Read the model definition and answer for the solid it produces. Units are mm, in the model's axes. A direction names the side the tool comes from. Coordinates: 2 decimals unless noted, no trailing zeros. Write each loop counter-clockwise with the first axis right and the second up, starting at its lowest first coordinate (ties: lowest second). Pieces come first, ordered by that corner, then holes. Notation, with made-up numbers: (89.25, 4.25) - (133.25, 4.25) arc R27 ccw to (133.25, 29.25) - close; hole circle Ø6 at (-22.75, -10.5). An arc over 180 degrees is marked (long way). Use a Markdown table: item, result.
from build123d import *

# Parameters (mm, degrees)
BOSS_EXTRUDE1_DEPTH = 3.9
SKETCH1_6_R         = 2.1
CUT_EXTRUDE1_DEPTH  = 1.6


with BuildPart() as part:
    # Sketch1 → Boss-Extrude1 (new body)
    with BuildSketch(Plane(origin=(0, 0, 0), x_dir=(1, 0, 0), z_dir=(0, 1, 0))):
        with BuildLine():
            Line((-105.9, 60.929794432), (-105.9, -60.929794385))
            ThreePointArc((-105.9, -60.929794385), (-105.050609665, -62.980404051), (-103, -63.829794385))
            Line((-103, -63.829794385), (2, -63.829794385))
            Line((2, -63.829794385), (2, 63.829794385))
            Line((2, 63.829794385), (-103, 63.829794385))
            ThreePointArc((-103, 63.829794385), (-105.050609649, 62.980404067), (-105.9, 60.929794432))
        make_face()
    extrude(amount=BOSS_EXTRUDE1_DEPTH)

    # Sketch1_6 → Cut-Extrude1 (cut)
    with BuildSketch(Plane(origin=(0, 0, 0), x_dir=(1, 0, 0), z_dir=(0, 1, 0))):
        with Locations(Location((-5, 60.929794385, 0), (0, 0, 270))):
            Circle(SKETCH1_6_R)
        with Locations(Location((-103, -60.929794385, 0), (0, 0, 270))):
            Circle(SKETCH1_6_R)
        with Locations(Location((-5, -60.929794385, 0), (0, 0, 270))):
            Circle(SKETCH1_6_R)
        with Locations(Location((-103, 60.929794385, 0), (0, 0, 270))):
            Circle(SKETCH1_6_R)
    extrude(amount=CUT_EXTRUDE1_DEPTH, mode=Mode.SUBTRACT)


solid = part.part
(1) Each of these flat-tipped pins is pushed along its axis until it touches: P1, Ø3.5, axis at x = -102, z = 61, coming from the -Y side; P2, Ø1.3, axis at x = -103, z = -61.5, coming from the -Y side. Where does it stop, or does it pass through?
Report:
| item | result |
|---|---|
| P1 | stops at y = 0 |
| P2 | stops at y = 1.6 |
(2) For faces 1 (the cylindrical face through (-6.278, 0.789, -62.596)), 2 (the flat face through (-53, 0, -1)), determine the directions among +Z, -Z, +X, -X, +Y, -Y from which every point of the face is accessible in a straight line to the end or side of a thin tool.
Report:
| item | result |
|---|---|
| face 1 | -Y |
| face 2 | +Z, -Z, +X, -X, -Y |
(3) A cutting plane is placed at A-A, the plane x = -5. Write down the section's boundary in (y, z).
Report:
| item | result |
|---|---|
| outline | (0, -63.83) - (3.9, -63.83) - (3.9, 63.83) - (0, 63.83) - (0, 63.03) - (1.6, 63.03) - (1.6, 58.83) - (0, 58.83) - (0, -58.83) - (1.6, -58.83) - (1.6, -63.03) - (0, -63.03) - close |
(4) The mould has two halves that part along Z. Classify faces 3 (the flat face through (-5, 1.6, 61)), 4 (the flat face through (-51, 2, 63.83)), 5 (the flat face through (-105.9, 2, -1)): pulls with the +Z half, pulls with the -Z half, needs draft (parallel to the pull), parting line crosses it, or undercut.
Report:
| item | result |
|---|---|
| face 3 | undercut |
| face 4 | pulls with the +Z half |
| face 5 | needs draft |
